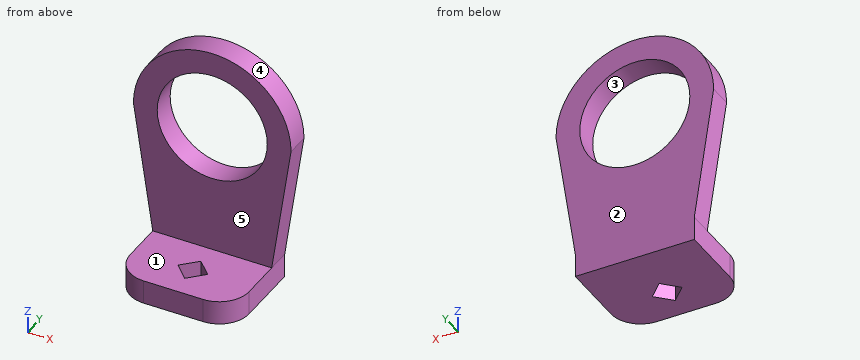
from build123d import *

# Parameters (mm, degrees)
F1_DEPTH = 16
F0_R     = 9.25
F2_DEPTH = 4
F4_R     = 5
F5_DEPTH = 4


with BuildPart() as f1:
    # F0 (on Front) → F1 (new body)
    with BuildSketch(Plane.XZ):
        Polygon((-10, 0), (0, 0), (10, 0), (10, 4), (0, 4), (-10, 4), align=None)
    extrude(amount=F1_DEPTH)

    # F0 (on Front) → F2 (join)
    with BuildSketch(Plane.XZ):
        with BuildLine():
            Line((-13.25, 26), (-10, 4))
            Line((-10, 4), (0, 4))
            Line((0, 4), (10, 4))
            Line((10, 4), (13.25, 26))
            ThreePointArc((13.25, 26), (0, 39.25), (-13.25, 26))
        make_face()
        with Locations((0, 26)):
            Circle(F0_R, mode=Mode.SUBTRACT)
    extrude(amount=F2_DEPTH)

    # F4
    f4_edges = [f1.edges().sort_by_distance(p)[0] for p in [
        (-10, -16, 2),
        (10, -16, 2),
    ]]
    fillet(f4_edges, radius=F4_R)

    # F3 (on face) → F5 (cut)
    with BuildSketch(Plane.XY.offset(4)):
        Polygon((-2.5, -10), (0, -10), (0, -7.5), align=None)
        Polygon((0, -12.5), (0, -10), (-2.5, -10), align=None)
        Polygon((2.5, -10), (0, -10), (0, -12.5), align=None)
        Polygon((0, -7.5), (0, -10), (2.5, -10), align=None)
    extrude(amount=-F5_DEPTH, mode=Mode.SUBTRACT)


solid = f1.part
Verification items for the finished model (mm, model axes). Face numbers are marked on the shaded views. A direction names the side the tool comes from. Give positions to 0.01 mm unless a question says otherwise; leave off trailing zeros. Loops run counter-clockwise (first coordinate to the right, second up) from the corner with the lowest first, then second, coordinate; pieces in that order, holes last.
1. Material ranges on probe 1 along Z at (x, y) = (0, -3.05); probe 2 along Z at (x, y) = (6, -9.75); probe 3 along Y at (x, z) = (5.25, 10), recorded low to high.
Derived:
probe 1: z = 0 to 16.75, 35.25 to 39.25
probe 2: z = 0 to 4
probe 3: y = -4 to 0
2. Cross-section at D-D on y = -6. Record the cut outline in (x, z), and give its area (3 significant figures).
Derived:
outline: (-10, 0) - (10, 0) - (10, 4) - (-10, 4) - close
area: 80.0 mm2
3. Tool access check on the marked faces 4 and 5. Record the directions out of +Z, -Z, +X, -X, +Y, -Y that give a thin tool (end or side, any length) a straight path to the whole face; none if there is none.
Derived:
face 4: +Z, +Y, -Y
face 5: +Z, +X, -X, -Y
4. Cross-section at C-C on x = -4.5. Record the cut outline in (y, z), and give its area (3 significant figures).
Derived:
outline: (-16, 0) - (0, 0) - (0, 17.92) - (-4, 17.92) - (-4, 4) - (-16, 4) - close; (-4, 34.08) - (0, 34.08) - (0, 38.46) - (-4, 38.46) - close
area: 137 mm2
5. Go/stop test with flat-tipped pins: P1, Ø1.5, axis at x = -2.5, z = 17, coming from the -Y side; P2, Ø2, axis at y = -6.5, z = 1.5, coming from the -X side; P3, Ø3, axis at y = -3.5, z = 2.5, coming from the +X side. Record where each tip stops, or that it passes through.
Derived:
P1: stops at y = -4
P2: stops at x = -10
P3: stops at x = 10
6. Release check for a two-part mould opening along Z. For the marked faces 1, 2 and 3 record: +Z half, -Z half, draft (parallel to the pull), parting line (faces both ways), or undercut.
Derived:
face 1: +Z half
face 2: draft
face 3: undercut
7. Cross-section at A-A on z = 3.5. Record the cut outline in (x, y).
Derived:
outline: (-10, -11) arc R5 ccw to (-5, -16) - (5, -16) arc R5 ccw to (10, -11) - (10, 0) - (-10, 0) - close; hole (-2.5, -10) - (0, -12.5) - (2.5, -10) - (0, -7.5) - close
8. Cross-section at B-B on x = 1.5. Record the cut outline in (y, z).
Derived:
outline: (-16, 0) - (-11, 0) - (-11, 4) - (-16, 4) - close; (-9, 0) - (0, 0) - (0, 16.87) - (-4, 16.87) - (-4, 4) - (-9, 4) - close; (-4, 35.13) - (0, 35.13) - (0, 39.16) - (-4, 39.16) - close
